Check sheet for the modelled part. Datum: model origin and axes. Units: mm. A direction names the side the tool comes from. Give positions to 0.01 mm unless a question says otherwise; leave off trailing zeros. Order: outer loops, then holes, each group sorted by start corner. A loop starts at its lowest first (then second) coordinate and runs counter-clockwise, first axis right, second up. Notation, with made-up numbers: (68, 57.25) - (83, 57.25) arc R18 cw to (83, 62.25) - close; hole circle Ø6 at (57, 2). An arc over 180 degrees is marked (long way). Answer in a Markdown table with one row per item.
from build123d import *

# Parameters (mm, degrees)
F0_W     = 20
F0_H     = 20
F1_DEPTH = 20
F2_W     = 16
F2_H     = 16
F3_DEPTH = 15
F4_W     = 16
F4_H     = 16
F5_DEPTH = 15
F6_W     = 16
F6_H     = 16
F7_DEPTH = 15
F8_W     = 16
F8_H     = 16
F9_DEPTH = 15


with BuildPart() as f1:
    # F0 (on Front) → F1 (new body)
    with BuildSketch(Plane.XZ):
        with Locations((10, -10)):
            Rectangle(F0_W, F0_H)
    extrude(amount=F1_DEPTH)

    # F2 (on face) → F3 (join)
    with BuildSketch(Plane.XY):
        with Locations((10, -10)):
            Rectangle(F2_W, F2_H)
    extrude(amount=F3_DEPTH)

    # F4 (on face) → F5 (join)
    with BuildSketch(Plane(origin=(0, 0, 0), x_dir=(-1, 0, 0), z_dir=(0, 1, 0))):
        with Locations((-10, -10)):
            Rectangle(F4_W, F4_H)
    extrude(amount=F5_DEPTH)

    # F6 (on face) → F7 (join)
    with BuildSketch(Plane.YZ.offset(20)):
        with Locations((-10, -10)):
            Rectangle(F6_W, F6_H)
    extrude(amount=F7_DEPTH)

    # F8 (on face) → F9 (join)
    with BuildSketch(Plane.XZ.offset(20)):
        with Locations((10, -10)):
            Rectangle(F8_W, F8_H)
    extrude(amount=F9_DEPTH)


solid = f1.part
(1) Cross-section at C-C, the plane x = 3.5. Record the cut outline in (y, z).
Geometry says:
| item | result |
|---|---|
| outline | (-35, -18) - (-20, -18) - (-20, -20) - (0, -20) - (0, -18) - (15, -18) - (15, -2) - (0, -2) - (0, 0) - (-2, 0) - (-2, 15) - (-18, 15) - (-18, 0) - (-20, 0) - (-20, -2) - (-35, -2) - close |
(2) Mould release check, pull along Z, two halves, no side actions. Record for faces 4 (the flat face through (10, 7, -18)), 5 (the flat face through (18, -10, 7)), 6 (the flat face through (10, -10, 15)): pulls with the +Z half, pulls with the -Z half, needs draft (parallel to the pull), parting line crosses it, or undercut.
Geometry says:
| item | result |
|---|---|
| face 4 | pulls with the -Z half |
| face 5 | needs draft |
| face 6 | pulls with the +Z half |
(3) Gauge pin test, flat ends, axial feed: P1, Ø3, axis at x = 16, z = 11.5, coming from the +Y side; P2, Ø4, axis at x = 17.5, y = -21.5, coming from the +Z side; P3, Ø4.5, axis at x = 28, z = -13, coming from the -Y side; P4, Ø3, axis at x = 23, y = -21.5, coming from the -Z side. Record the tip position at first contact, or that the pin passes through.
Geometry says:
| item | result |
|---|---|
| P1 | y = -2 |
| P2 | z = 0 |
| P3 | y = -18 |
| P4 | through |
(4) Cross-section at A-A, the plane z = -7.5. Record the cut outline in (x, y).
Geometry says:
| item | result |
|---|---|
| outline | (0, -20) - (2, -20) - (2, -35) - (18, -35) - (18, -20) - (20, -20) - (20, -18) - (35, -18) - (35, -2) - (20, -2) - (20, 0) - (18, 0) - (18, 15) - (2, 15) - (2, 0) - (0, 0) - close |
(5) Thickness scan on L1, parallel to Z at x = 15.5, y = -29; L2, parallel to X at y = -18.5, z = -7. Record the ranges inside material, lowest first.
Geometry says:
| item | result |
|---|---|
| L1 | -18 to -2 |
| L2 | 0 to 20 |
(6) Access from +Z, -Z, +X, -X, +Y, -Y to the whole of each face (thin tool, end or side, straight path). Record for faces 1 (the flat face through (18, 7, -10)), 2 (the flat face through (10, -27, -2)), 3 (the flat face through (2, -10, 7)).
Geometry says:
| item | result |
|---|---|
| face 1 | +Z, -Z, +X, +Y |
| face 2 | +Z, +X, -X, -Y |
| face 3 | +Z, -X, +Y, -Y |
(7) Cross-section at B-B, the plane y = -3. Record the cut outline in (x, z).
Geometry says:
| item | result |
|---|---|
| outline | (0, -20) - (20, -20) - (20, -18) - (35, -18) - (35, -2) - (20, -2) - (20, 0) - (18, 0) - (18, 15) - (2, 15) - (2, 0) - (0, 0) - close |
(8) Cross-section at D-D, the plane z = 9. Record the cut outline in (x, y), then the cut area to 3 significant figures.
Geometry says:
| item | result |
|---|---|
| outline | (2, -18) - (18, -18) - (18, -2) - (2, -2) - close |
| area | 256 mm² |
